The listing builds one solid part. Answer for the finished solid, in the listing's coordinates (mm). Coordinates: 2 decimals unless noted, no trailing zeros. Loops run counter-clockwise (first coordinate to the right, second up) from the corner with the lowest first, then second, coordinate; pieces in that order, holes last. Notation, with made-up numbers: (8.25, 13.25) -> (49.25, 13.25) arc R14 ccw to (49.25, 39.25) -> close; hole circle Ø1 at (29, -3). An arc over 180 degrees is marked (long way). Answer in a Markdown table with one row per item.
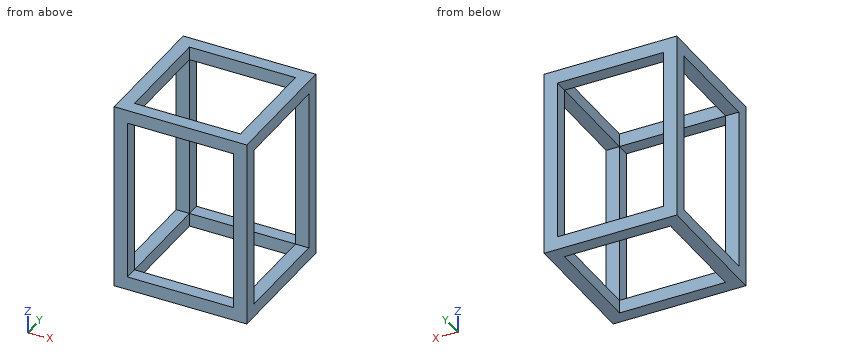
Autodesk Inventor part; units mm, degrees
ref_plane "YZ Plane" through (0, 0, 0) normal (1, 0, 0) x (0, 1, 0)
ref_plane "XZ Plane" through (0, 0, 0) normal (0, 1, 0) x (-1, 0, 0)
ref_plane "XY Plane" through (0, 0, 0) normal (0, 0, 1) x (1, 0, 0)
sketch "Sketch1" plane through (0, 0, 0) normal (0, 0, 1) x (1, 0, 0)
  line L0 (0, 0) -> (200, 0)
  line L1 (200, 0) -> (200, 196.27)
  line L2 (200, 196.27) -> (0, 196.27)
  line L3 (0, 196.27) -> (0, 0)
  dimension "d0" = 200
  dimension "d1" = 196.27
extrude "Extrusion1" add sketch "Sketch1" along normal blind 284.3
sketch "Sketch2" plane through (0, 0, 284.3) normal (0, 0, 1) x (1, 0, 0)
  line L0 (20, 176.27) -> (180, 176.27)
  line L1 (180, 176.27) -> (180, 20)
  line L2 (180, 20) -> (20, 20)
  line L3 (20, 20) -> (20, 176.27)
  line L4 (200, 196.27) -> (0, 196.27)
  line L5 (0, 196.27) -> (0, 0)
  line L6 (200, 0) -> (200, 196.27)
  line L7 (0, 0) -> (200, 0)
  dimension "d4" = 20
  dimension "d5" = 20
  dimension "d6" = 20
  dimension "d7" = 20
extrude "Extrusion2" cut sketch "Sketch2" against normal blind 900 contours L0 L1 L2 L3
sketch "Sketch3" plane through (200, 0, 0) normal (1, 0, 0) x (0, 0, -1)
  line L0 (-264.3, 176.27) -> (-20, 176.27)
  line L1 (-20, 176.27) -> (-20, 20)
  line L2 (-20, 20) -> (-264.3, 20)
  line L3 (-264.3, 20) -> (-264.3, 176.27)
  line L4 (0, 196.27) -> (-284.3, 196.27)
  line L5 (-284.3, 0) -> (-284.3, 196.27)
  line L6 (0, 0) -> (-284.3, 0)
  line L7 (0, 0) -> (0, 196.27)
  dimension "d10" = 20
  dimension "d11" = 20
  dimension "d12" = 20
  dimension "d13" = 20
extrude "Extrusion3" cut sketch "Sketch3" against normal blind 900 contours L0 L1 L2 L3
sketch "Sketch4" plane through (0, 196.27, 0) normal (0, 1, 0) x (1, 0, 0)
  line L0 (20, -264.3) -> (0, -264.3)
  line L1 (180, -20) -> (180, 0)
  line L2 (20, -264.3) -> (180, -264.3)
  line L3 (180, -264.3) -> (180, -20)
  line L4 (180, -20) -> (20, -20)
  line L5 (20, -20) -> (20, -264.3)
  point P0 (0, 0)
extrude "Extrusion4" cut sketch "Sketch4" against normal blind 900
properties part number "Motor Pump Housing"
Item 1: Find the intervals of material crossed by probe 1 along Z at (x, y) = (87, 13.5); probe 2 along X at (y, z) = (14.5, 55.5); probe 3 along Y at (x, z) = (165, 264.5), in increasing order.
Findings below:
| item | result |
|---|---|
| probe 1 | z = 0 to 20, 264.3 to 284.3 |
| probe 2 | x = 0 to 20, 180 to 200 |
| probe 3 | y = 0 to 20, 176.27 to 196.27 |
Item 2: A cutting plane is placed at C-C, the plane y = 121. Determine the outline of the cut face in (x, z).
Findings below:
| item | result |
|---|---|
| outline | (0, 0) -> (20, 0) -> (20, 20) -> (0, 20) -> close; (0, 264.3) -> (20, 264.3) -> (20, 284.3) -> (0, 284.3) -> close; (180, 0) -> (200, 0) -> (200, 20) -> (180, 20) -> close; (180, 264.3) -> (200, 264.3) -> (200, 284.3) -> (180, 284.3) -> close |
Item 3: A cutting plane is placed at A-A, the plane x = 80.5. Determine the outline of the cut face in (y, z), plus the area to 3 significant figures.
Findings below:
| item | result |
|---|---|
| outline | (0, 0) -> (20, 0) -> (20, 20) -> (0, 20) -> close; (0, 264.3) -> (20, 264.3) -> (20, 284.3) -> (0, 284.3) -> close; (176.27, 0) -> (196.27, 0) -> (196.27, 20) -> (176.27, 20) -> close; (176.27, 264.3) -> (196.27, 264.3) -> (196.27, 284.3) -> (176.27, 284.3) -> close |
| area | 1,600 mm2 |
Item 4: A cutting plane is placed at B-B, the plane y = 181. Determine the outline of the cut face in (x, z).
Findings below:
| item | result |
|---|---|
| outline | (0, 0) -> (200, 0) -> (200, 284.3) -> (0, 284.3) -> close; hole (20, 20) -> (180, 20) -> (180, 264.3) -> (20, 264.3) -> close |
